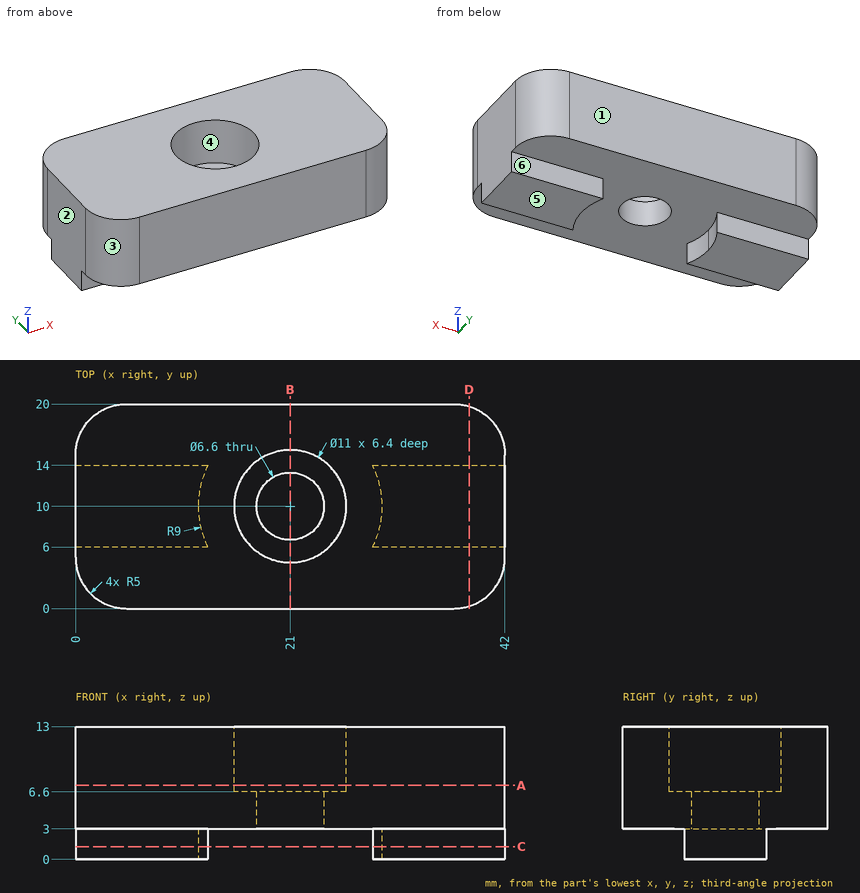
Check sheet for the drawn part. Datum: minimum x, y, z corner. Units: mm. A direction names the side the tool comes from. Give positions to 0.01 mm unless a question says otherwise; leave off trailing zeros. Write each loop counter-clockwise with the first axis right and the second up, starting at its lowest first coordinate (ties: lowest second). Pieces come first, ordered by that corner, then holes. Notation, with made-up numbers: M 35.5,59.5 L 64.5,59.5 A34 cw 64.5,91.5 Z; hole C 43.5,-4 d10. An arc over 180 degrees is marked long. Write item = value, one per line.
(1) Access from +Z, -Z, +X, -X, +Y, -Y to the whole of each face (thin tool, end or side, straight path). Record for the marked faces 5 and 6.
Found:
face_5 = -Z, +X, -X, +Y, -Y
face_6 = -Z, +X, -X, +Y
(2) Sectioned sample at C-C (z = 1.25). Record the cut outline in (x, y).
Found:
outline = M 0,6 L 12.94,6 A9 cw 12.94,14 L 0,14 Z; M 29.06,6 L 42,6 L 42,14 L 29.06,14 A9 cw Z
(3) Material ranges on line 1 (Y direction, x = 21, z = 9.5); line 2 (Y direction, x = 21, z = 5.35); line 3 (X direction, y = 8, z = 12.5), recorded low to high.
Found:
line_1 = 0 to 4.5, 15.5 to 20
line_2 = 0 to 6.7, 13.3 to 20
line_3 = 0 to 15.88, 26.12 to 42
(4) Sectioned sample at B-B (x = 21). Record the cut outline in (y, z).
Found:
outline = M 0,3 L 6.7,3 L 6.7,6.6 L 4.5,6.6 L 4.5,13 L 0,13 Z; M 13.3,3 L 20,3 L 20,13 L 15.5,13 L 15.5,6.6 L 13.3,6.6 Z
(5) Draft check along Y on the marked faces 1, 2, 3 and 4. Enter one of: released by +Y, released by -Y, zero draft, split by the parting line, or undercut.
Found:
face_1 = released by +Y
face_2 = zero draft
face_3 = released by -Y
face_4 = undercut
(6) Go/stop test with flat-tipped pins: pin 1 Ø12 at (x, y) = (23, 7.5) entering from +Z; pin 2 Ø4 at (x, y) = (23.5, 9.5) entering from +Z; pin 3 Ø1.5 at (x, y) = (21.5, 4) entering from -Z; pin 4 Ø0.9 at (x, z) = (32.5, 1.5) entering from -Y. Record where each tip stops, or that it passes through.
Found:
pin_1 = 13
pin_2 = 6.6
pin_3 = 3
pin_4 = 6
(7) Sectioned sample at A-A (z = 7.25). Record the cut outline in (x, y).
Found:
outline = M 0,5 A5 ccw 5,0 L 37,0 A5 ccw 42,5 L 42,15 A5 ccw 37,20 L 5,20 A5 ccw 0,15 Z; hole C 21,10 d11
(8) Sectioned sample at D-D (x = 38.5). Record the cut outline in (y, z), then the cut area to 3 significant figures.
Found:
outline = M 0.23,3 L 6,3 L 6,0 L 14,0 L 14,3 L 19.77,3 L 19.77,13 L 0.23,13 Z
area = 219 mm2
